Autodesk Inventor part; units mm, degrees
ref_plane "YZ Plane" through (0, 0, 0) normal (1, 0, 0) x (0, 1, 0)
ref_plane "XZ Plane" through (0, 0, 0) normal (0, 1, 0) x (-1, 0, 0)
ref_plane "XY Plane" through (0, 0, 0) normal (0, 0, 1) x (1, 0, 0)
sketch "Sketch1" plane through (0, 0, 0) normal (0, 0, 1) x (1, 0, 0)
  line L0 (-250, -250) -> (250, -250)
  line L1 (250, -250) -> (250, 250)
  line L2 (250, 250) -> (-250, 250)
  line L3 (-250, 250) -> (-250, -250)
  line L4 (-250, -250) -> (250, 250) construction
  line L5 (250, -250) -> (-250, 250) construction
  point P0 (0, 0)
  dimension "d0" = 500
  dimension "d1" = 500
extrude "Extrusion1" add sketch "Sketch1" along normal blind 1.5875
sketch "Sketch2" plane through (0, 0, 1.5875) normal (0, 0, 1) x (1, 0, 0)
  line L0 (-250, -250) -> (250, -250)
  line L1 (250, -250) -> (250, 250)
  line L2 (250, 250) -> (-250, 250)
  line L3 (-250, 250) -> (-250, -250)
  point P0 (0, 0)
  point P1 (-220, 240)
  dimension "d4" = 10
  dimension "d5" = 30
hole "Hole1" at (-220, 240, 1.5875) direction (0, 0, -1) diameter 5 end through all
pattern_linear "Rectangular Pattern1" count 5 spacing 110 along (1, 0, 0) count 2 spacing 480 along (0, -1, 0) of "Hole1"
sketch "Sketch3" plane through (0, 0, 1.5875) normal (0, 0, 1) x (1, 0, 0)
  circle A0 centre (220, -240) radius 2.5
  circle A1 centre (110, -240) radius 2.5
  circle A2 centre (0, -240) radius 2.5
  circle A3 centre (-110, -240) radius 2.5
  circle A4 centre (-220, -240) radius 2.5
  circle A5 centre (220, 240) radius 2.5
  circle A6 centre (110, 240) radius 2.5
  circle A7 centre (0, 240) radius 2.5
  circle A8 centre (-110, 240) radius 2.5
  circle A9 centre (-220, 240) radius 2.5
  line L0 (-250, -250) -> (250, -250)
  line L1 (250, -250) -> (250, 250)
  line L2 (250, 250) -> (-250, 250)
  line L3 (-250, 250) -> (-250, -250)
  point P0 (0, 0)
  point P1 (-240, 220)
  dimension "d19" = 10
  dimension "d20" = 30
hole "Hole2" at (-240, 220, 1.5875) direction (0, 0, -1) diameter 5 end through all
pattern_linear "Rectangular Pattern2" count 5 spacing 110 along (0, -1, 0) count 2 spacing 480 along (1, 0, 0) of "Hole2"
properties part number "Face B Felt" material "Nylon 6/6"
The model under review builds one solid part; all positions refer to its coordinate system, in mm. Round coordinates to 2 decimals unless told otherwise and drop trailing zeros.
Item 1: For line 1 (Y direction, x = -240, z = 0.8); line 2 (Y direction, x = 0, z = 0.6), list the stretches that pass through material, from the lowest coordinate up.
Determined:
line 1: y = -250 to -222.5, -217.5 to -112.5, -107.5 to -2.5, 2.5 to 107.5, 112.5 to 217.5, 222.5 to 250
line 2: y = -250 to -242.5, -237.5 to 237.5, 242.5 to 250
Item 2: Mouldability with a two-part tool opening along Z and no side actions: class faces 1 (the face through (-3, 4, 1.588)), 2 (the face through (-3, 4, 0)) as released by +Z, released by -Z, zero draft, split by the parting line, or undercut.
Determined:
face 1: released by +Z
face 2: released by -Z
Item 3: Clearance check with flat-ended pins moving along their axes: pin 1 Ø8 at (x, y) = (110, -240) entering from -Z; pin 2 Ø4 at (x, y) = (0, 240) entering from +Z. State where each tip first meets the part, or that it passes through.
Determined:
pin 1: stops at z = 0
pin 2: passes through
